Read the model definition and answer for the solid it produces. Units are mm, in the model's axes. A direction names the side the tool comes from. Coordinates: 2 decimals unless noted, no trailing zeros. Loops run counter-clockwise (first coordinate to the right, second up) from the corner with the lowest first, then second, coordinate; pieces in that order, holes last. Notation, with made-up numbers: (-34, -22) -> (-18, -22) arc R17 ccw to (-18, -14) -> close; hole circle Ø10 at (80.25, -21.5). An arc over 180 degrees is marked (long way). Answer in a Markdown table with one row per item.
```python
from build123d import *

# Parameters (mm, degrees)
F1_DEPTH = 13
F2_DEPTH = 25
F3_W     = 110
F3_H     = 15
F4_DEPTH = 25
F5_DEPTH = 25
F6_R     = 12.5
F7_DEPTH = 25


with BuildPart() as f1:
    # F0 (on Front) → F1 (new body)
    with BuildSketch(Plane.XZ):
        with BuildLine():
            Line((112.3251678944, 210), (-144.6748321056, 210))
            ThreePointArc((-144.6748321056, 210), (-158.8169677293, 204.1421356237), (-164.6748321056, 190))
            Line((-164.6748321056, 190), (-164.6748321056, 20))
            ThreePointArc((-164.6748321056, 20), (-158.8169677293, 5.8578643763), (-144.6748321056, 0))
            Line((-144.6748321056, 0), (112.3251678944, 0))
            ThreePointArc((112.3251678944, 0), (126.4673035181, 5.8578643763), (132.3251678944, 20))
            Line((132.3251678944, 20), (132.3251678944, 190))
            ThreePointArc((132.3251678944, 190), (126.4673035181, 204.1421356237), (112.3251678944, 210))
        make_face()
    extrude(amount=F1_DEPTH)

    # F0 (on Front) + F1_face (on face) → F2 (join)
    with BuildSketch(Plane.XZ):
        with BuildLine():
            Line((112.3251678944, 210), (-144.6748321056, 210))
            ThreePointArc((-144.6748321056, 210), (-158.8169677293, 204.1421356237), (-164.6748321056, 190))
            Line((-164.6748321056, 190), (-164.6748321056, 20))
            ThreePointArc((-164.6748321056, 20), (-158.8169677293, 5.8578643763), (-144.6748321056, 0))
            Line((-144.6748321056, 0), (112.3251678944, 0))
            ThreePointArc((112.3251678944, 0), (126.4673035181, 5.8578643763), (132.3251678944, 20))
            Line((132.3251678944, 20), (132.3251678944, 190))
            ThreePointArc((132.3251678944, 190), (126.4673035181, 204.1421356237), (112.3251678944, 210))
        make_face()
    with BuildSketch(Plane(origin=(-16.1748321056, -13, 105), x_dir=(1, 0, 0), z_dir=(0, -1, 0))):
        with BuildLine():
            Line((148.5, -85), (148.5, 85))
            ThreePointArc((148.5, 85), (142.6421356237, 99.1421356237), (128.5, 105))
            Line((128.5, 105), (-128.5, 105))
            ThreePointArc((-128.5, 105), (-142.6421356237, 99.1421356237), (-148.5, 85))
            Line((-148.5, 85), (-148.5, -85))
            ThreePointArc((-148.5, -85), (-142.6421356237, -99.1421356237), (-128.5, -105))
            Line((-128.5, -105), (128.5, -105))
            ThreePointArc((128.5, -105), (142.6421356237, -99.1421356237), (148.5, -85))
        make_face()
    extrude(amount=F2_DEPTH)

    # F3 (on face) → F4 (cut)
    with BuildSketch(Plane.XZ.offset(38)):
        with Locations((98.1996059418, 165.9660535473)):
            Rectangle(F3_W, F3_H)
    extrude(amount=-F4_DEPTH, mode=Mode.SUBTRACT)

    # F5 (cut): a face of the model
    f5_faces = [f1.faces().sort_by_distance(p)[0] for p in [
        (87.7623869181, -13, 165.9660535473),
    ]]
    extrude(f5_faces, amount=-F5_DEPTH, mode=Mode.SUBTRACT)

    # F6 (on face) → F7 (join)
    with BuildSketch(Plane.XZ.offset(38)):
        with BuildLine():
            ThreePointArc((-164.6748321056, 20), (-158.8169677293, 5.8578643763), (-144.6748321056, 0))
            Line((-144.6748321056, 0), (112.3251678944, 0))
            ThreePointArc((112.3251678944, 0), (126.4673035181, 5.8578643763), (132.3251678944, 20))
            Line((132.3251678944, 20), (132.3251678944, 158.4660535473))
            Line((132.3251678944, 158.4660535473), (43.1996059418, 158.4660535473))
            Line((43.1996059418, 158.4660535473), (43.1996059418, 173.4660535473))
            Line((43.1996059418, 173.4660535473), (132.3251678944, 173.4660535473))
            Line((132.3251678944, 173.4660535473), (132.3251678944, 190))
            ThreePointArc((132.3251678944, 190), (126.4673035181, 204.1421356237), (112.3251678944, 210))
            Line((112.3251678944, 210), (-144.6748321056, 210))
            ThreePointArc((-144.6748321056, 210), (-158.8169677293, 204.1421356237), (-164.6748321056, 190))
            Line((-164.6748321056, 190), (-164.6748321056, 20))
        make_face()
        with Locations((2.5, 72.5)):
            Circle(F6_R, mode=Mode.SUBTRACT)
        with Locations((57.5, 72.5)):
            Circle(F6_R, mode=Mode.SUBTRACT)
        with Locations((112.5, 72.5)):
            Circle(F6_R, mode=Mode.SUBTRACT)
        with Locations((2.5, 72.5)):
            Circle(F6_R)
        with Locations((57.5, 72.5)):
            Circle(F6_R)
    extrude(amount=F7_DEPTH)


solid = f1.part
```
1. The mould has two halves that part along Z. Classify faces 1 (the cylindrical face through (126.31, -31.06, 5.7)), 2 (the flat face through (87, -31, 173.466)), 3 (the flat face through (-164.675, -31, 106)), 4 (the cylindrical face through (124.423, -50.325, 76.255)): pulls with the +Z half, pulls with the -Z half, needs draft (parallel to the pull), parting line crosses it, or undercut.
A:
| item | result |
|---|---|
| face 1 | pulls with the -Z half |
| face 2 | undercut |
| face 3 | needs draft |
| face 4 | undercut |
2. A cutting plane is placed at D-D on z = 72.5. Give the vertices of the cut face in (x, y).
A:
| item | result |
|---|---|
| outline | (-164.67, -63) -> (100, -63) -> (100, -38) -> (125, -38) -> (125, -63) -> (132.33, -63) -> (132.33, 0) -> (-164.67, 0) -> close |
3. Find the intervals of material crossed by probe 1 along Z at (x, y) = (112.5, -45); probe 2 along Z at (x, y) = (93, -16.5); probe 3 along X at (y, z) = (-55, 72), in increasing order.
A:
| item | result |
|---|---|
| probe 1 | z = 0 to 60, 85 to 158.47, 173.47 to 210 |
| probe 2 | z = 0 to 158.47, 173.47 to 210 |
| probe 3 | x = -164.67 to 100.01, 124.99 to 132.33 |
4. Given pin 1 Ø22.5 at (x, z) = (112.5, 72.5) entering from -Y, flat-ended and moving along its own axis, determine where the tip first touches the part or whether it passes through.
A:
| item | result |
|---|---|
| pin 1 | stops at y = -38 |
5. A cutting plane is placed at A-A on x = 75. Give the vertices of the cut face in (y, z).
A:
| item | result |
|---|---|
| outline | (-63, 0) -> (0, 0) -> (0, 158.47) -> (-63, 158.47) -> close; (-63, 173.47) -> (0, 173.47) -> (0, 210) -> (-63, 210) -> close |
6. A cutting plane is placed at B-B on y = -53. Give the vertices of the cut face in (x, z), and give its area (3 significant figures).
A:
| item | result |
|---|---|
| outline | (-164.67, 20) arc R20 ccw to (-144.67, 0) -> (112.33, 0) arc R20 ccw to (132.33, 20) -> (132.33, 158.47) -> (43.2, 158.47) -> (43.2, 173.47) -> (132.33, 173.47) -> (132.33, 190) arc R20 ccw to (112.33, 210) -> (-144.67, 210) arc R20 ccw to (-164.67, 190) -> close; hole circle Ø25 at (112.5, 72.5) |
| area | 60,200 mm2 |
7. A cutting plane is placed at C-C on y = -29. Give the vertices of the cut face in (x, z).
A:
| item | result |
|---|---|
| outline | (-164.67, 20) arc R20 ccw to (-144.67, 0) -> (112.33, 0) arc R20 ccw to (132.33, 20) -> (132.33, 158.47) -> (43.2, 158.47) -> (43.2, 173.47) -> (132.33, 173.47) -> (132.33, 190) arc R20 ccw to (112.33, 210) -> (-144.67, 210) arc R20 ccw to (-164.67, 190) -> close |
8. A tool of negligible diameter and unlimited length cuts with its end or side. For faces 5 (the flat face through (43.2, -31, 166)), 6 (the flat face through (112, -38, 73)), 7 (the flat face through (132.325, -31, 182)), from which of +Z, -Z, +X, -X, +Y, -Y can it reach the whole face along a straight path? Write none if from no direction.
A:
| item | result |
|---|---|
| face 5 | +X, +Y, -Y |
| face 6 | -Y |
| face 7 | +Z, -Z, +X, +Y, -Y |
